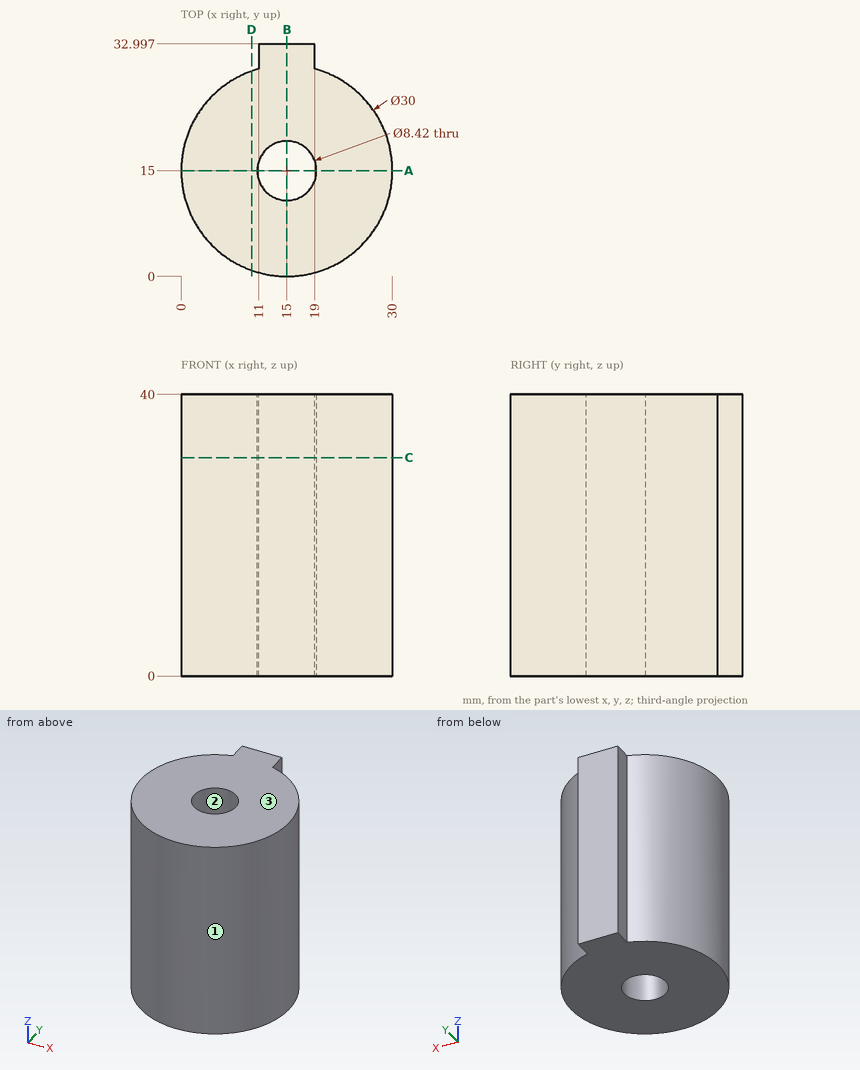
Source: three-view drawing plus pictorial views. Frame: mm from the lowest corner of the part. Coordinates: 2 decimals unless noted, no trailing zeros. Order: outer loops, then holes, each group sorted by start corner. A loop starts at its lowest first (then second) coordinate and runs counter-clockwise, first axis right, second up. Notation, with made-up numbers: M 40,43.5 L 87,43.5 A4 ccw 87,48.5 Z; hole C 36,-32.5 d5. An arc over 180 degrees is marked long. Write each question's results on one line, items separated by ' | '. Start each with the question number.
1. Draft query along Y for the marked faces 1, 2 and 3. Return one class per face: +Y half, -Y half, draft (parallel to the pull), parting line (faces both ways), or undercut.
2. Pin query (flat end, axial travel): pin 1 (3 mm diameter, centred on y = 31.5, z = 12, fed in from +X); pin 2 (5 mm diameter, centred on y = 6.5, z = 22.5, fed in from +X); pin 3 (1.8 mm diameter, centred on y = 31.5, z = 18, fed in from -X). Return the tip coordinate at first contact, or that it passes through.
3. Section A-A, the plane y = 15. Return the cut outline in (x, z), then the cut area to 3 significant figures.
4. Material intervals for L1, parallel to Y at x = 12, z = 20.5; L2, parallel to X at y = 17.5, z = 30; L3, parallel to Y at x = 26.5, z = 2.5, sorted ascending.
5. Section C-C, the plane z = 31. Return the cut outline in (x, y).
6. Section D-D, the plane x = 10. Return the cut outline in (y, z).
7. Section B-B, the plane x = 15. Return the cut outline in (y, z), then the cut area to 3 significant figures.
Solution:
1) face 1: parting line | face 2: undercut | face 3: draft
2) pin 1: x = 19 | pin 2: x = 28.75 | pin 3: x = 11
3) outline: M 0,0 L 10.79,0 L 10.79,40 L 0,40 Z; M 19.21,0 L 30,0 L 30,40 L 19.21,40 Z | area: 863 mm²
4) L1: 0.3 to 12.05, 17.95 to 33 | L2: 0.21 to 11.61, 18.39 to 29.79 | L3: 5.37 to 24.63
5) outline: M 11,29.46 A15 ccw long 19,29.46 L 19,33 L 11,33 Z; hole C 15,15 d8.42
6) outline: M 0.86,0 L 29.14,0 L 29.14,40 L 0.86,40 Z
7) outline: M 0,0 L 10.79,0 L 10.79,40 L 0,40 Z; M 19.21,0 L 33,0 L 33,40 L 19.21,40 Z | area: 983 mm²
